Verification items for the finished model (mm, model axes). Face numbers are marked on the shaded views. A direction names the side the tool comes from. Give positions to 0.01 mm unless a question says otherwise; leave off trailing zeros. Order: outer loops, then holes, each group sorted by start corner. A loop starts at its lowest first (then second) coordinate and runs counter-clockwise, first axis right, second up. Notation, with made-up numbers: (73, 47) - (83, 47) arc R6 cw to (83, 56) - close; hole circle Ø3 at (61.25, 85.25). An arc over 180 degrees is marked (long way). Answer as a JSON object with one key per item and string values. Group by question number.
(1) Access from +Z, -Z, +X, -X, +Y, -Y to the whole of each face (thin tool, end or side, straight path). Record for the marked faces 1 and 2.
(2) Section check B-B (x = 46.5). Record the boundary of the cut face in (y, z).
(3) Thickness scan on line 1 (Z direction, x = -27, y = 43.5); line 2 (Y direction, x = -2, z = 2); line 3 (Z direction, x = -52.5, y = 1). Record the ranges inside material, lowest first.
(4) Section check C-C (y = 85). Record the boundary of the cut face in (x, z), then the cut area to 3 significant figures.
(5) Depth check by flat-ended pin: pin 1 Ø2 at (x, y) = (-50.8, 78.31) entering from -Z; pin 2 Ø3 at (x, z) = (8, -16) entering from +Y; pin 3 Ø2.5 at (x, y) = (0, 14.81) entering from -Z; pin 4 Ø2 at (x, z) = (35, 38.5) entering from -Y. Enter the tip coordinate at first touch or a pass-through.
(6) Section check A-A (z = -26). Record the boundary of the cut face in (x, y).
(7) Section check D-D (x = 15.5). Record the boundary of the cut face in (y, z).
```python
from build123d import *

# Parameters (mm, degrees)
SKETCH3_R                  = 2.65
BASE_FLANGE1_DEPTH         = 6.35
F_4_40_TAPPED_HOLE1_D      = 2.2606
LPATTERN1_COUNT            = 9
LPATTERN1_PITCH            = 12.7
LPATTERN1_COUNT_DIR2       = 9
LPATTERN1_PITCH_DIR2       = 12.7
SKETCHED_START             = 47.102289028
SKETCHED_BEND1_OUTLINE_W   = 127
SKETCHED_BEND1_OUTLINE_H   = 6.35
SKETCHED_BEND1_DEPTH       = 119.686790972
SKETCHED_START_2           = 35.707087028
SKETCHED_BEND1_2_OUTLINE_W = 127
SKETCHED_BEND1_2_OUTLINE_H = 124.066087028
SKETCHED_BEND1_2_OUTLINE_R = 1.1303
SKETCHED_BEND1_2_DEPTH     = 12.7
SKETCHED_START_3           = -63.5
SKETCHED_BEND1_3_DEPTH     = 127


with BuildPart() as part:
    # Base-Flange1: sheet metal written as solids
    # Sketch3 → Base-Flange1 (new body)
    with BuildSketch(Plane(origin=(0, 0, 0), x_dir=(1, 0, 0), z_dir=(0, 1, 0))):
        with BuildLine():
            Line((-63.5, -28.481), (-63.5, -166.78908))
            Line((-63.5, -166.78908), (63.5, -166.78908))
            Line((63.5, -166.78908), (63.5, -28.481))
            Line((63.5, -28.481), (35.019, 0))
            ThreePointArc((35.019, 0), (0, 35.019), (-35.019, 0))
            Line((-35.019, 0), (-63.5, -28.481))
        make_face()
        with Locations(Location((0, 25.019, 0), (0, 0, 270))):
            Circle(SKETCH3_R, mode=Mode.SUBTRACT)
        with Locations(Location((21.667089577, 12.5095, 0), (0, 0, 270))):
            Circle(SKETCH3_R, mode=Mode.SUBTRACT)
        with Locations(Location((21.667089577, -12.5095, 0), (0, 0, 270))):
            Circle(SKETCH3_R, mode=Mode.SUBTRACT)
        with Locations(Location((0, -25.019, 0), (0, 0, 270))):
            Circle(SKETCH3_R, mode=Mode.SUBTRACT)
        with Locations(Location((-21.667089577, -12.5095, 0), (0, 0, 270))):
            Circle(SKETCH3_R, mode=Mode.SUBTRACT)
        with Locations(Location((-21.667089577, 12.5095, 0), (0, 0, 270))):
            Circle(SKETCH3_R, mode=Mode.SUBTRACT)
    extrude(amount=-BASE_FLANGE1_DEPTH)

    # #4-40 Tapped Hole1 (through all)
    with Locations(Plane(origin=(-50.8, 0, 57.531), x_dir=(0, 0, 1), z_dir=(0, 1, 0))):
        with Locations((0, 0)):
            f_4_40_tapped_hole1 = Hole(F_4_40_TAPPED_HOLE1_D / 2)

    # LPattern1: 4-40 Tapped Hole1 9 × 9
    with Locations(*[(i * LPATTERN1_PITCH, 0, j * LPATTERN1_PITCH_DIR2) for i in range(LPATTERN1_COUNT) for j in range(LPATTERN1_COUNT_DIR2) if (i, j) != (0, 0)]):
        add(f_4_40_tapped_hole1, mode=Mode.SUBTRACT)

    # Sketched Bend1: read off the stored shape, not the designer's step
    # Sketched Bend1 outline → Sketched Bend1 (cut)
    with BuildSketch(Plane.XY.offset(SKETCHED_START)):
        with Locations((0, -3.175)):
            Rectangle(SKETCHED_BEND1_OUTLINE_W, SKETCHED_BEND1_OUTLINE_H)
    extrude(amount=SKETCHED_BEND1_DEPTH, mode=Mode.SUBTRACT)

    # Sketched Bend1 2 outline → Sketched Bend1 2 (add)
    with BuildSketch(Plane.XY.offset(SKETCHED_START_2)):
        with Locations((0, 62.033043514)):
            Rectangle(SKETCHED_BEND1_2_OUTLINE_W, SKETCHED_BEND1_2_OUTLINE_H)
        with Locations((-50.8, 14.808007028)):
            Circle(SKETCHED_BEND1_2_OUTLINE_R, mode=Mode.SUBTRACT)
        with Locations((-38.1, 14.808007028)):
            Circle(SKETCHED_BEND1_2_OUTLINE_R, mode=Mode.SUBTRACT)
        with Locations((-25.4, 14.808007028)):
            Circle(SKETCHED_BEND1_2_OUTLINE_R, mode=Mode.SUBTRACT)
        with Locations((-12.7, 14.808007028)):
            Circle(SKETCHED_BEND1_2_OUTLINE_R, mode=Mode.SUBTRACT)
        with Locations((-50.8, 27.508007028)):
            Circle(SKETCHED_BEND1_2_OUTLINE_R, mode=Mode.SUBTRACT)
        with Locations((-50.8, 40.208007028)):
            Circle(SKETCHED_BEND1_2_OUTLINE_R, mode=Mode.SUBTRACT)
        with Locations((-38.1, 27.508007028)):
            Circle(SKETCHED_BEND1_2_OUTLINE_R, mode=Mode.SUBTRACT)
        with Locations((-38.1, 40.208007028)):
            Circle(SKETCHED_BEND1_2_OUTLINE_R, mode=Mode.SUBTRACT)
        with Locations((-50.8, 52.908007028)):
            Circle(SKETCHED_BEND1_2_OUTLINE_R, mode=Mode.SUBTRACT)
        with Locations((-38.1, 52.908007028)):
            Circle(SKETCHED_BEND1_2_OUTLINE_R, mode=Mode.SUBTRACT)
        with Locations((-25.4, 27.508007028)):
            Circle(SKETCHED_BEND1_2_OUTLINE_R, mode=Mode.SUBTRACT)
        with Locations((-25.4, 40.208007028)):
            Circle(SKETCHED_BEND1_2_OUTLINE_R, mode=Mode.SUBTRACT)
        with Locations((-12.7, 27.508007028)):
            Circle(SKETCHED_BEND1_2_OUTLINE_R, mode=Mode.SUBTRACT)
        with Locations((-12.7, 40.208007028)):
            Circle(SKETCHED_BEND1_2_OUTLINE_R, mode=Mode.SUBTRACT)
        with Locations((-25.4, 52.908007028)):
            Circle(SKETCHED_BEND1_2_OUTLINE_R, mode=Mode.SUBTRACT)
        with Locations((-12.7, 52.908007028)):
            Circle(SKETCHED_BEND1_2_OUTLINE_R, mode=Mode.SUBTRACT)
        with Locations((0, 14.808007028)):
            Circle(SKETCHED_BEND1_2_OUTLINE_R, mode=Mode.SUBTRACT)
        with Locations((12.7, 14.808007028)):
            Circle(SKETCHED_BEND1_2_OUTLINE_R, mode=Mode.SUBTRACT)
        with Locations((25.4, 14.808007028)):
            Circle(SKETCHED_BEND1_2_OUTLINE_R, mode=Mode.SUBTRACT)
        with Locations((38.1, 14.808007028)):
            Circle(SKETCHED_BEND1_2_OUTLINE_R, mode=Mode.SUBTRACT)
        with Locations((50.8, 14.808007028)):
            Circle(SKETCHED_BEND1_2_OUTLINE_R, mode=Mode.SUBTRACT)
        with Locations((0, 27.508007028)):
            Circle(SKETCHED_BEND1_2_OUTLINE_R, mode=Mode.SUBTRACT)
        with Locations((12.7, 27.508007028)):
            Circle(SKETCHED_BEND1_2_OUTLINE_R, mode=Mode.SUBTRACT)
        with Locations((0, 40.208007028)):
            Circle(SKETCHED_BEND1_2_OUTLINE_R, mode=Mode.SUBTRACT)
        with Locations((12.7, 40.208007028)):
            Circle(SKETCHED_BEND1_2_OUTLINE_R, mode=Mode.SUBTRACT)
        with Locations((25.4, 27.508007028)):
            Circle(SKETCHED_BEND1_2_OUTLINE_R, mode=Mode.SUBTRACT)
        with Locations((25.4, 40.208007028)):
            Circle(SKETCHED_BEND1_2_OUTLINE_R, mode=Mode.SUBTRACT)
        with Locations((0, 52.908007028)):
            Circle(SKETCHED_BEND1_2_OUTLINE_R, mode=Mode.SUBTRACT)
        with Locations((12.7, 52.908007028)):
            Circle(SKETCHED_BEND1_2_OUTLINE_R, mode=Mode.SUBTRACT)
        with Locations((25.4, 52.908007028)):
            Circle(SKETCHED_BEND1_2_OUTLINE_R, mode=Mode.SUBTRACT)
        with Locations((38.1, 27.508007028)):
            Circle(SKETCHED_BEND1_2_OUTLINE_R, mode=Mode.SUBTRACT)
        with Locations((38.1, 40.208007028)):
            Circle(SKETCHED_BEND1_2_OUTLINE_R, mode=Mode.SUBTRACT)
        with Locations((50.8, 27.508007028)):
            Circle(SKETCHED_BEND1_2_OUTLINE_R, mode=Mode.SUBTRACT)
        with Locations((50.8, 40.208007028)):
            Circle(SKETCHED_BEND1_2_OUTLINE_R, mode=Mode.SUBTRACT)
        with Locations((38.1, 52.908007028)):
            Circle(SKETCHED_BEND1_2_OUTLINE_R, mode=Mode.SUBTRACT)
        with Locations((50.8, 52.908007028)):
            Circle(SKETCHED_BEND1_2_OUTLINE_R, mode=Mode.SUBTRACT)
        with Locations((-50.8, 65.608007028)):
            Circle(SKETCHED_BEND1_2_OUTLINE_R, mode=Mode.SUBTRACT)
        with Locations((-38.1, 65.608007028)):
            Circle(SKETCHED_BEND1_2_OUTLINE_R, mode=Mode.SUBTRACT)
        with Locations((-50.8, 78.308007028)):
            Circle(SKETCHED_BEND1_2_OUTLINE_R, mode=Mode.SUBTRACT)
        with Locations((-50.8, 91.008007028)):
            Circle(SKETCHED_BEND1_2_OUTLINE_R, mode=Mode.SUBTRACT)
        with Locations((-38.1, 78.308007028)):
            Circle(SKETCHED_BEND1_2_OUTLINE_R, mode=Mode.SUBTRACT)
        with Locations((-38.1, 91.008007028)):
            Circle(SKETCHED_BEND1_2_OUTLINE_R, mode=Mode.SUBTRACT)
        with Locations((-25.4, 65.608007028)):
            Circle(SKETCHED_BEND1_2_OUTLINE_R, mode=Mode.SUBTRACT)
        with Locations((-12.7, 65.608007028)):
            Circle(SKETCHED_BEND1_2_OUTLINE_R, mode=Mode.SUBTRACT)
        with Locations((-25.4, 78.308007028)):
            Circle(SKETCHED_BEND1_2_OUTLINE_R, mode=Mode.SUBTRACT)
        with Locations((-25.4, 91.008007028)):
            Circle(SKETCHED_BEND1_2_OUTLINE_R, mode=Mode.SUBTRACT)
        with Locations((-12.7, 78.308007028)):
            Circle(SKETCHED_BEND1_2_OUTLINE_R, mode=Mode.SUBTRACT)
        with Locations((-12.7, 91.008007028)):
            Circle(SKETCHED_BEND1_2_OUTLINE_R, mode=Mode.SUBTRACT)
        with Locations((-50.8, 103.708007028)):
            Circle(SKETCHED_BEND1_2_OUTLINE_R, mode=Mode.SUBTRACT)
        with Locations((-38.1, 103.708007028)):
            Circle(SKETCHED_BEND1_2_OUTLINE_R, mode=Mode.SUBTRACT)
        with Locations((-50.8, 116.408007028)):
            Circle(SKETCHED_BEND1_2_OUTLINE_R, mode=Mode.SUBTRACT)
        with Locations((-38.1, 116.408007028)):
            Circle(SKETCHED_BEND1_2_OUTLINE_R, mode=Mode.SUBTRACT)
        with Locations((-25.4, 103.708007028)):
            Circle(SKETCHED_BEND1_2_OUTLINE_R, mode=Mode.SUBTRACT)
        with Locations((-12.7, 103.708007028)):
            Circle(SKETCHED_BEND1_2_OUTLINE_R, mode=Mode.SUBTRACT)
        with Locations((-25.4, 116.408007028)):
            Circle(SKETCHED_BEND1_2_OUTLINE_R, mode=Mode.SUBTRACT)
        with Locations((-12.7, 116.408007028)):
            Circle(SKETCHED_BEND1_2_OUTLINE_R, mode=Mode.SUBTRACT)
        with Locations((0, 65.608007028)):
            Circle(SKETCHED_BEND1_2_OUTLINE_R, mode=Mode.SUBTRACT)
        with Locations((12.7, 65.608007028)):
            Circle(SKETCHED_BEND1_2_OUTLINE_R, mode=Mode.SUBTRACT)
        with Locations((25.4, 65.608007028)):
            Circle(SKETCHED_BEND1_2_OUTLINE_R, mode=Mode.SUBTRACT)
        with Locations((0, 78.308007028)):
            Circle(SKETCHED_BEND1_2_OUTLINE_R, mode=Mode.SUBTRACT)
        with Locations((12.7, 78.308007028)):
            Circle(SKETCHED_BEND1_2_OUTLINE_R, mode=Mode.SUBTRACT)
        with Locations((0, 91.008007028)):
            Circle(SKETCHED_BEND1_2_OUTLINE_R, mode=Mode.SUBTRACT)
        with Locations((12.7, 91.008007028)):
            Circle(SKETCHED_BEND1_2_OUTLINE_R, mode=Mode.SUBTRACT)
        with Locations((25.4, 78.308007028)):
            Circle(SKETCHED_BEND1_2_OUTLINE_R, mode=Mode.SUBTRACT)
        with Locations((25.4, 91.008007028)):
            Circle(SKETCHED_BEND1_2_OUTLINE_R, mode=Mode.SUBTRACT)
        with Locations((38.1, 65.608007028)):
            Circle(SKETCHED_BEND1_2_OUTLINE_R, mode=Mode.SUBTRACT)
        with Locations((50.8, 65.608007028)):
            Circle(SKETCHED_BEND1_2_OUTLINE_R, mode=Mode.SUBTRACT)
        with Locations((38.1, 78.308007028)):
            Circle(SKETCHED_BEND1_2_OUTLINE_R, mode=Mode.SUBTRACT)
        with Locations((38.1, 91.008007028)):
            Circle(SKETCHED_BEND1_2_OUTLINE_R, mode=Mode.SUBTRACT)
        with Locations((50.8, 78.308007028)):
            Circle(SKETCHED_BEND1_2_OUTLINE_R, mode=Mode.SUBTRACT)
        with Locations((50.8, 91.008007028)):
            Circle(SKETCHED_BEND1_2_OUTLINE_R, mode=Mode.SUBTRACT)
        with Locations((0, 103.708007028)):
            Circle(SKETCHED_BEND1_2_OUTLINE_R, mode=Mode.SUBTRACT)
        with Locations((12.7, 103.708007028)):
            Circle(SKETCHED_BEND1_2_OUTLINE_R, mode=Mode.SUBTRACT)
        with Locations((25.4, 103.708007028)):
            Circle(SKETCHED_BEND1_2_OUTLINE_R, mode=Mode.SUBTRACT)
        with Locations((0, 116.408007028)):
            Circle(SKETCHED_BEND1_2_OUTLINE_R, mode=Mode.SUBTRACT)
        with Locations((12.7, 116.408007028)):
            Circle(SKETCHED_BEND1_2_OUTLINE_R, mode=Mode.SUBTRACT)
        with Locations((25.4, 116.408007028)):
            Circle(SKETCHED_BEND1_2_OUTLINE_R, mode=Mode.SUBTRACT)
        with Locations((38.1, 103.708007028)):
            Circle(SKETCHED_BEND1_2_OUTLINE_R, mode=Mode.SUBTRACT)
        with Locations((50.8, 103.708007028)):
            Circle(SKETCHED_BEND1_2_OUTLINE_R, mode=Mode.SUBTRACT)
        with Locations((38.1, 116.408007028)):
            Circle(SKETCHED_BEND1_2_OUTLINE_R, mode=Mode.SUBTRACT)
        with Locations((50.8, 116.408007028)):
            Circle(SKETCHED_BEND1_2_OUTLINE_R, mode=Mode.SUBTRACT)
    extrude(amount=SKETCHED_BEND1_2_DEPTH)

    # Sketched Bend1 3 outline → Sketched Bend1 3 (cut)
    with BuildSketch(Plane.YZ.offset(SKETCHED_START_3)):
        with BuildLine():
            ThreePointArc((-6.35, 35.707087028), (-2.630256121, 44.687343149), (6.35, 48.407087028))
            Line((6.35, 48.407087028), (0, 48.407087028))
            Line((0, 48.407087028), (0, 47.102289028))
            Line((0, 47.102289028), (-6.35, 47.102289028))
            Line((-6.35, 47.102289028), (-6.35, 35.707087028))
        make_face()
        with BuildLine():
            Line((124.066087028, 42.057087028), (6.35, 42.057087028))
            ThreePointArc((6.35, 42.057087028), (1.859871939, 40.197215088), (0, 35.707087028))
            Line((0, 35.707087028), (124.066087028, 35.707087028))
            Line((124.066087028, 35.707087028), (124.066087028, 42.057087028))
        make_face()
    extrude(amount=SKETCHED_BEND1_3_DEPTH, mode=Mode.SUBTRACT)


solid = part.part
```
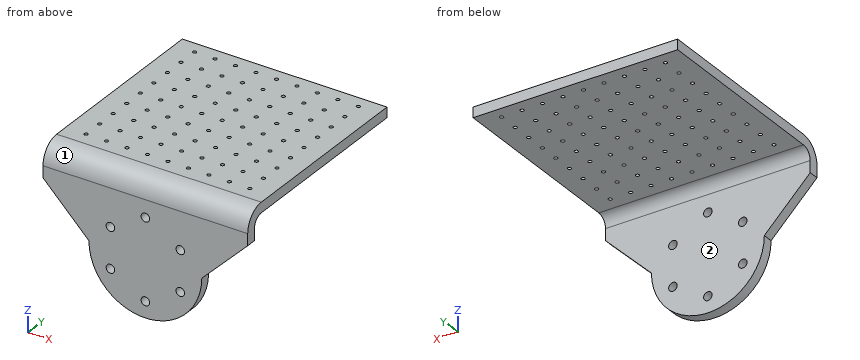
Solutions:
{
 "1": {"face 1": "+Z, +X, -X, -Y", "face 2": "-Z, +X, -X, +Y"},
 "2": {"outline": "(-6.35, 11.48) - (0, 11.48) - (0, 35.71) arc R6.35 cw to (6.35, 42.06) - (124.07, 42.06) - (124.07, 48.41) - (6.35, 48.41) arc R12.7 ccw to (-6.35, 35.71) - close"},
 "3": {"line 1": "z = 42.06 to 48.41", "line 2": "y = -6.35 to 0", "line 3": "z = 39.13 to 47.23"},
 "4": {"outline": "(-63.5, 42.06) - (63.5, 42.06) - (63.5, 48.41) - (-63.5, 48.41) - close", "area": "806 mm2"},
 "5": {"pin 1": "passes through", "pin 2": "stops at y = 0", "pin 3": "stops at z = 42.06", "pin 4": "stops at y = -6.22"},
 "6": {"outline": "(-23.46, -6.35) - (-2.46, -6.35) - (-2.46, 0) - (-23.46, 0) - close; (2.46, -6.35) - (23.46, -6.35) - (23.46, 0) - (2.46, 0) - close"},
 "7": {"outline": "(-6.35, -31.4) - (0, -31.4) - (0, 35.71) arc R6.35 cw to (6.35, 42.06) - (124.07, 42.06) - (124.07, 48.41) - (6.35, 48.41) arc R12.7 ccw to (-6.35, 35.71) - close"}
}
